from build123d import *

# Parameters (mm, degrees)
SKETCH1_W          = 12.7
SKETCH1_H          = 20.574
EXTRUDE1_DEPTH     = 1.5875
SKETCH3_R          = 1.5875
CUT_EXTRUDE6_DEPTH = 13.192826795
CIRPATTERN1_COUNT  = 2
SKETCH5_R          = 2.5
CUT_EXTRUDE8_DEPTH = 13.192826795


with BuildPart() as part:
    # Sketch1 → Extrude1 (new body)
    with BuildSketch(Plane(origin=(0, 0, 0), x_dir=(1, 0, 0), z_dir=(0, 1, 0))):
        Rectangle(SKETCH1_W, SKETCH1_H)
    extrude(amount=EXTRUDE1_DEPTH)

    # Sketch3 → Cut-Extrude6 (cut, through all)
    with BuildSketch(Plane(origin=(0, 0, 0), x_dir=(1, 0, 0), z_dir=(0, 1, 0))):
        with Locations(Location((0, 7.14375, 0), (0, 0, 270))):
            Circle(SKETCH3_R)
    cut_extrude6 = extrude(amount=CUT_EXTRUDE6_DEPTH, mode=Mode.SUBTRACT)

    # CirPattern1: Cut-Extrude6 ×2 about axis
    cirpattern1_axis = Axis((0, 0, 0), (0, 1, 0))
    for i in range(1, CIRPATTERN1_COUNT):
        add(cut_extrude6.rotate(cirpattern1_axis, i * 360 / CIRPATTERN1_COUNT), mode=Mode.SUBTRACT)

    # Sketch5 → Cut-Extrude8 (cut, through all)
    with BuildSketch(Plane(origin=(0, 0, 0), x_dir=(1, 0, 0), z_dir=(0, 1, 0))):
        with Locations(Location((0, 0, 0), (0, 0, 270))):
            Circle(SKETCH5_R)
    extrude(amount=CUT_EXTRUDE8_DEPTH, mode=Mode.SUBTRACT)


solid = part.part
The model under review builds one solid part; all positions refer to its coordinate system, in mm. Coordinates: 2 decimals unless noted, no trailing zeros. Write each loop counter-clockwise with the first axis right and the second up, starting at its lowest first coordinate (ties: lowest second). Pieces come first, ordered by that corner, then holes. Notation, with made-up numbers: (11, 58.25) -> (49, 58.25) arc R15 cw to (49, 65.25) -> close; hole circle Ø2 at (-32.75, 6). An arc over 180 degrees is marked (long way). Answer in a Markdown table with one row per item.
1. We need section C-C, the plane y = 0.45. Give the number of separate pieces and of enclosed holes in the cut face, and give its area (3 significant figures).
Answers below:
| item | result |
|---|---|
| separate pieces | 1 |
| enclosed holes | 3 |
| area | 226 mm^2 |
2. We need section B-B, the plane x = 0. State the section outline as (y, z) points.
Answers below:
| item | result |
|---|---|
| outline | (0, -10.29) -> (1.59, -10.29) -> (1.59, -8.73) -> (0, -8.73) -> close; (0, -5.56) -> (1.59, -5.56) -> (1.59, -2.5) -> (0, -2.5) -> close; (0, 2.5) -> (1.59, 2.5) -> (1.59, 5.56) -> (0, 5.56) -> close; (0, 8.73) -> (1.59, 8.73) -> (1.59, 10.29) -> (0, 10.29) -> close |
3. We need section D-D, the plane z = -6. State the section outline as (x, y) points, and give its area (3 significant figures).
Answers below:
| item | result |
|---|---|
| outline | (-6.35, 0) -> (-1.1, 0) -> (-1.1, 1.59) -> (-6.35, 1.59) -> close; (1.1, 0) -> (6.35, 0) -> (6.35, 1.59) -> (1.1, 1.59) -> close |
| area | 16.7 mm^2 |
4. Clearance check with a flat-ended pin moving along its axis: pin 1 Ø1.9 at (x, z) = (0, -7.14) entering from +Y. State where the tip first meets the part, or that it passes through.
Answers below:
| item | result |
|---|---|
| pin 1 | passes through |
5. Wall thickness on probe 1 along Z at (x, y) = (0, 0.45); probe 2 along X at (y, z) = (0.75, 0); probe 3 along Z at (x, y) = (1, 1.3): over which ranges is each line inside the solid? List them lowest first. Write a range as [from, to].
Answers below:
| item | result |
|---|---|
| probe 1 | z = [-10.29, -8.73], [-5.56, -2.5], [2.5, 5.56], [8.73, 10.29] |
| probe 2 | x = [-6.35, -2.5], [2.5, 6.35] |
| probe 3 | z = [-10.29, -8.38], [-5.91, -2.29], [2.29, 5.91], [8.38, 10.29] |
6. Draft analysis for pull direction Z (two halves, no side actions). For faces 1 (the flat face through (6.35, 1, 0)), 2 (the flat face through (0, 1, -10.287)), 3 (the cylindrical face through (-2.44, 0.78, -0.54)), state which applies: +Z half, -Z half, draft (parallel to the pull), parting line (faces both ways), or undercut.
Answers below:
| item | result |
|---|---|
| face 1 | draft |
| face 2 | -Z half |
| face 3 | undercut |
7. We need section A-A, the plane z = 0. State the section outline as (x, y) points, and give its area (3 significant figures).
Answers below:
| item | result |
|---|---|
| outline | (-6.35, 0) -> (-2.5, 0) -> (-2.5, 1.59) -> (-6.35, 1.59) -> close; (2.5, 0) -> (6.35, 0) -> (6.35, 1.59) -> (2.5, 1.59) -> close |
| area | 12.2 mm^2 |
